from build123d import *

# Parameters (mm, degrees)
SKETCH1_R           = 160
SKETCH1_R_2         = 1.5
BOSS_EXTRUDE1_DEPTH = 5


with BuildPart() as part:
    # Sketch1 → Boss-Extrude1 (new body)
    with BuildSketch(Plane(origin=(0, 0, 0), x_dir=(1, 0, 0), z_dir=(0, 1, 0))):
        with Locations(Location((0, 0, 0), (0, 0, 270))):
            Circle(SKETCH1_R)
        with Locations(Location((155, 0, 0), (0, 0, 270))):
            Circle(SKETCH1_R_2, mode=Mode.SUBTRACT)
        with Locations(Location((0, -155, 0), (0, 0, 270))):
            Circle(SKETCH1_R_2, mode=Mode.SUBTRACT)
        with Locations(Location((-155, 0, 0), (0, 0, 270))):
            Circle(SKETCH1_R_2, mode=Mode.SUBTRACT)
        with Locations(Location((0, 155, 0), (0, 0, 270))):
            Circle(SKETCH1_R_2, mode=Mode.SUBTRACT)
        Polygon((7.505553499, 0), (3.75277675, 6.5), (-3.75277675, 6.5), (-7.505553499, 0), (-3.75277675, -6.5), (3.75277675, -6.5), align=None, mode=Mode.SUBTRACT)
    extrude(amount=-BOSS_EXTRUDE1_DEPTH)


solid = part.part
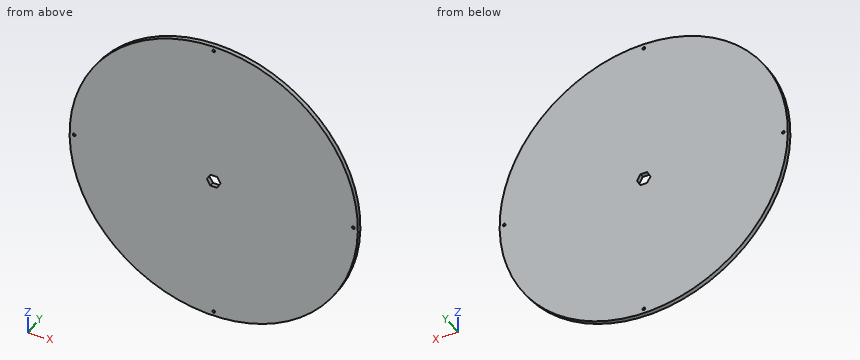
CAD build for the part. Positions are in the model's coordinates, mm. Round coordinates to 2 decimals unless told otherwise and drop trailing zeros. Loops run counter-clockwise (first coordinate to the right, second up) from the corner with the lowest first, then second, coordinate; pieces in that order, holes last. Notation, with made-up numbers: M 34,86 L 48,86 A14 cw 48,105 Z; hole C -20.5,-20.5 d4. An arc over 180 degrees is marked long. One line per question, with ' | ' between items. Start each with the question number.
Item 1: Cut at C-C, the plane z = 137.5. Write the cut outline in (x, y).
Item 2: Wall check: line 1 (X direction, y = -1.6, z = 0); line 2 (X direction, y = -4.2, z = -72.5); line 3 (X direction, y = -0.7, z = -10). Give the ranges that are in metal, low to high.
Item 3: Pin check, flat tips, straight feed: pin 1 Ø4 at (x, z) = (0, -155) entering from +Y; pin 2 Ø2 at (y, z) = (-1, 123) entering from -X; pin 3 Ø1 at (y, z) = (-2.5, -80.5) entering from +X. Stop position of each tip, or through.
Item 4: Cut at A-A, the plane y = -4.1. Write the cut outline in (x, z).
Item 5: Cut at B-B, the plane x = 40. Write the cut outline in (y, z), plus the area to 3 significant figures.
Responses:
1) outline: M -81.82,-5 L 81.82,-5 L 81.82,0 L -81.82,0 Z
2) line 1: x = -160 to -156.5, -153.5 to -7.51, 7.51 to 153.5, 156.5 to 160 | line 2: x = -142.63 to 142.63 | line 3: x = -159.69 to 159.69
3) pin 1: stops at y = 0 | pin 2: stops at x = -103.52 | pin 3: stops at x = 138.56
4) outline: C 0,0 d320; hole C -155,0 d3; hole M -7.51,0 L -3.75,-6.5 L 3.75,-6.5 L 7.51,0 L 3.75,6.5 L -3.75,6.5 Z; hole C 0,-155 d3; hole C 0,155 d3; hole C 155,0 d3
5) outline: M -5,-154.92 L 0,-154.92 L 0,154.92 L -5,154.92 Z | area: 1,550 mm²
